```python
from build123d import *

# Parameters (mm, degrees)
F0_W      = 9.9
F0_H      = 9.9
F1_DEPTH  = 20
F3_DEPTH  = 9.901
F5_DEPTH  = 9.901
F6_R      = 2.65
F7_DEPTH  = 20.001
F9_DEPTH  = 3
F10_START = -3
F10_DEPTH = 0.2


with BuildPart() as f1:
    # F0 (on Front) → F1 (new body)
    with BuildSketch(Plane.XZ):
        Rectangle(F0_W, F0_H)
    extrude(amount=F1_DEPTH)

    # F2 (on face) → F3 (cut, through all)
    with BuildSketch(Plane(origin=(0, 0, -4.95), x_dir=(1, 0, 0), z_dir=(0, 0, -1))):
        Polygon((-4.95, 7.6), (-4.95, 5.6), (-3.95, 5.6), align=None)
        Polygon((-4.95, 10.6), (-4.95, 8.6), (-3.95, 8.6), align=None)
        Polygon((-4.95, 13.6), (-4.95, 11.6), (-3.95, 11.6), align=None)
        Polygon((-4.95, 16.6), (-4.95, 14.6), (-3.95, 14.6), align=None)
        Polygon((-3.95, 17.6), (-4.95, 19.6), (-4.95, 17.6), align=None)
        Polygon((4.95, 5.6), (4.95, 7.6), (3.95, 5.6), align=None)
        Polygon((3.95, 8.6), (4.95, 8.6), (4.95, 10.6), align=None)
        Polygon((3.95, 11.6), (4.95, 11.6), (4.95, 13.6), align=None)
        Polygon((3.95, 14.6), (4.95, 14.6), (4.95, 16.6), align=None)
        Polygon((3.95, 17.6), (4.95, 17.6), (4.95, 19.6), align=None)
    extrude(amount=-F3_DEPTH, mode=Mode.SUBTRACT)

    # F4 (on face) → F5 (cut, through all)
    with BuildSketch(Plane.YZ.offset(4.95)):
        Polygon((10.1219329327, 0.5148088664), (10.1219329327, 2.5148088664), (9.1219329327, 0.5148088664), align=None)
        Polygon((-5.6, 3.95), (-5.6, 4.95), (-7.6, 4.95), align=None)
        Polygon((-8.6, 4.95), (-10.6, 4.95), (-8.6, 3.95), align=None)
        Polygon((-11.6, 4.95), (-13.6, 4.95), (-11.6, 3.95), align=None)
        Polygon((-14.6, 4.95), (-16.6, 4.95), (-14.6, 3.95), align=None)
        Polygon((-10.6, -4.95), (-8.6, -4.95), (-8.6, -3.95), align=None)
        Polygon((-16.6, -4.95), (-14.6, -4.95), (-14.6, -3.95), align=None)
        Polygon((-7.6, -4.95), (-5.6, -4.95), (-5.6, -3.95), align=None)
        Polygon((-13.6, -4.95), (-11.6, -4.95), (-11.6, -3.95), align=None)
        Polygon((-17.6, 4.95), (-19.6, 4.95), (-17.6, 3.95), align=None)
        Polygon((-17.6, -4.95), (-17.6, -3.95), (-19.6, -4.95), align=None)
    extrude(amount=-F5_DEPTH, mode=Mode.SUBTRACT)

    # F6 (on face) → F7 (cut, through all)
    with BuildSketch(Plane(origin=(0, 0, 0), x_dir=(-1, 0, 0), z_dir=(0, 1, 0))):
        Circle(F6_R)
    extrude(amount=-F7_DEPTH, mode=Mode.SUBTRACT)

    # F8 (on face) → F9 (cut)
    with BuildSketch(Plane(origin=(0, 0, 0), x_dir=(-1, 0, 0), z_dir=(0, 1, 0))):
        Polygon((0, -4.5), (3.897114317, -2.25), (3.897114317, 2.25), (0, 4.5), (-3.897114317, 2.25), (-3.897114317, -2.25), align=None)
    extrude(amount=-F9_DEPTH, mode=Mode.SUBTRACT)

    # F8 (on face) → F10 (join)
    with BuildSketch(Plane(origin=(0, 0, 0), x_dir=(-1, 0, 0), z_dir=(0, 1, 0)).offset(F10_START)):
        Polygon((0, -4.5), (3.897114317, -2.25), (3.897114317, 2.25), (0, 4.5), (-3.897114317, 2.25), (-3.897114317, -2.25), align=None)
    extrude(amount=-F10_DEPTH)


solid = f1.part
```
Geometry: final body of the model. Coordinates: model frame, mm. A direction names the side the tool comes from. Give positions to 0.01 mm unless a question says otherwise; leave off trailing zeros. Loops run counter-clockwise (first coordinate to the right, second up) from the corner with the lowest first, then second, coordinate; pieces in that order, holes last. Notation, with made-up numbers: (29.5, 70) -> (56.5, 70) arc R27 ccw to (56.5, 96) -> close; hole circle Ø11 at (71.5, 2). An arc over 180 degrees is marked (long way). Use one line per item in the form item = value.
Item 1: Line query: probe 1 along Z at (x, y) = (0, -11); probe 2 along Y at (x, z) = (-3.5, 4.5); probe 3 along X at (y, z) = (-1, 1.25). Output: solid intervals per line, ascending.
A:
probe_1 = -4.95 to -2.65, 2.65 to 4.95
probe_2 = -20 to -18.7, -17.6 to -15.7, -14.6 to -12.7, -11.6 to -9.7, -8.6 to -6.7, -5.6 to 0
probe_3 = -4.95 to -3.9, 3.9 to 4.95
Item 2: Section query B-B on y = -4.75. Output: boundary loops of the cut face in (x, z), and give its area (3 significant figures).
A:
outline = (-4.95, -4.95) -> (4.95, -4.95) -> (4.95, 4.95) -> (-4.95, 4.95) -> close; hole circle Ø5.3 at (0, 0)
area = 75.9 mm^2
Item 3: Section query A-A on x = -4.5. Give the number of separate pieces and of enclosed holes in the cut face, and give its area (3 significant figures).
A:
separate_pieces = 6
enclosed_holes = 0
area = 142 mm^2
Item 4: Draft query along Y for faces 1 (the face through (4.457, -6.614, -0.069)), 2 (the face through (0, -11, 4.95)). Return one class per face: pulls with the +Y half, pulls with the -Y half, needs draft (parallel to the pull), parting line crosses it, or undercut.
A:
face_1 = undercut
face_2 = needs draft
Item 5: Section query C-C on y = -12.5. Output: boundary loops of the cut face in (x, z).
A:
outline = (-4.4, -4.4) -> (4.4, -4.4) -> (4.4, 4.4) -> (-4.4, 4.4) -> close; hole circle Ø5.3 at (0, 0)
Item 6: Access query for faces 3 (the face through (-4.443, -6.586, -0.069)), 4 (the face through (0.069, -12.586, -4.443)), 5 (the face through (4.457, -9.614, -0.069)), 6 (the face through (0.069, -6.614, 4.457)). Directions: +Z, -Z, +X, -X, +Y, -Y. A direction counts if a zero-diameter tool reaches every point of the face in a straight line with its end or side. Return the directions, or none.
A:
face_3 = +Z, -Z, -X
face_4 = -Z, +X, -X
face_5 = +Z, -Z, +X
face_6 = +Z, +X, -X
Item 7: Pin query (flat end, axial travel): P1, Ø1.6, axis at x = -0.5, z = -0.5, coming from the -Y side; P2, Ø4, axis at x = 0, z = -0.5, coming from the +Y side. Return the tip coordinate at first contact, or that it passes through.
A:
P1 = -3.2
P2 = -3
